from build123d import *

# Parameters (mm, degrees)
SKETCH_1_W          = 20
SKETCH_1_H          = 10.24
EXTRUDE_1_DEPTH     = 6.5
SKETCH_2_R          = 1.25
CUT_EXTRUDE_1_DEPTH = 7.5
SKETCH_4_W          = 2.303604444
SKETCH_4_H          = 2.775905185
EXTRUDE_2_DEPTH     = 8


with BuildPart() as part:
    # 草图1 → 凸台-拉伸1 (new body)
    with BuildSketch(Plane(origin=(0, 0, 0), x_dir=(1, 0, 0), z_dir=(0, 1, 0))):
        Rectangle(SKETCH_1_W, SKETCH_1_H)
    extrude(amount=EXTRUDE_1_DEPTH)

    # 草图2 → 切除-拉伸1 (cut, through all)
    with BuildSketch(Plane(origin=(0, 6.5, 0), x_dir=(1, 0, 0), z_dir=(0, 1, 0))):
        with Locations((-4.75, -2.62)):
            Circle(SKETCH_2_R)
        with Locations((4.75, -2.62)):
            Circle(SKETCH_2_R)
    extrude(amount=-CUT_EXTRUDE_1_DEPTH, mode=Mode.SUBTRACT)

    # 草图4 → 凸台-拉伸2 (add)
    with BuildSketch(Plane(origin=(0, 0, -5.12), x_dir=(-1, 0, 0), z_dir=(0, 0, -1))):
        with Locations((8.848197778, 3.213855402)):
            Rectangle(SKETCH_4_W, SKETCH_4_H)
    extrude(amount=EXTRUDE_2_DEPTH)


solid = part.part
Could you check a few things on this model? Use its own coordinates, in mm. A direction names the side the tool comes from. Coordinates: 2 decimals unless noted, no trailing zeros. Loops run counter-clockwise (first coordinate to the right, second up) from the corner with the lowest first, then second, coordinate; pieces in that order, holes last.
1. Imagine slicing it at A-A (x = -5.5). Please give me the cut outline in (y, z), and give its area (3 significant figures).
2. Imagine slicing it at B-B (z = 2.62). Please give me the cut outline in (x, y).
3. Imagine slicing it at D-D (x = 4.75). Please give me the cut outline in (y, z).
4. Imagine slicing it at C-C (y = 4). Please give me the cut outline in (x, z).
5. For faces 5 (the face through (-9, 4.602, -9)), 6 (the face through (-9, 1.826, -9)), 7 (the face through (-5.74, 3.3, 3.38)), 8 (the face through (-7.696, 3, -9)), which set-ups out of +Z, -Z, +X, -X, +Y, -Y let a thin tool reach every point of the face, with its end or its side?
6. We'd pull the mould along Z, two halves only. Please class faces 1 (the face through (4.48, 3.3, 3.84)), 2 (the face through (0, 3, 5.12)), 3 (the face through (0, 0, 0)), 4 (the face through (-9, 3, -13.12)): released by +Z, released by -Z, zero draft, split by the parting line, or undercut.
7. For P1, Ø1.5, axis at x = -2.5, y = 1, coming from the -Z side; P2, Ø0.8, axis at y = 3.5, z = -10, coming from the +X side; P3, Ø2.5, axis at x = -9, z = -9.5, coming from the -Y side, each with a flat end and sliding along its axis, tell me the tip position at first contact or that it passes through.
8. I need wall thicknesses on L1, parallel to X at y = 3.75, z = 2.62; L2, parallel to Z at x = 4.75, y = 2; L3, parallel to Z at x = 8.5, y = 1. Which ranges of each line are inside material? Lowest first, please.
Computed values:
1. outline: (0, -5.12) - (6.5, -5.12) - (6.5, 1.62) - (0, 1.62) - close; (0, 3.62) - (6.5, 3.62) - (6.5, 5.12) - (0, 5.12) - close
1. area: 53.6 mm2
2. outline: (-10, 0) - (-6, 0) - (-6, 6.5) - (-10, 6.5) - close; (-3.5, 0) - (3.5, 0) - (3.5, 6.5) - (-3.5, 6.5) - close; (6, 0) - (10, 0) - (10, 6.5) - (6, 6.5) - close
3. outline: (0, -5.12) - (6.5, -5.12) - (6.5, 1.37) - (0, 1.37) - close; (0, 3.87) - (6.5, 3.87) - (6.5, 5.12) - (0, 5.12) - close
4. outline: (-10, -13.12) - (-7.7, -13.12) - (-7.7, -5.12) - (10, -5.12) - (10, 5.12) - (-10, 5.12) - close; hole circle Ø2.5 at (-4.75, 2.62); hole circle Ø2.5 at (4.75, 2.62)
5. face 5: -Z, +X, -X, +Y
5. face 6: -Z, +X, -X, -Y
5. face 7: +Y, -Y
5. face 8: -Z, +X, +Y, -Y
6. face 1: undercut
6. face 2: released by +Z
6. face 3: zero draft
6. face 4: released by -Z
7. P1: stops at z = -5.12
7. P2: stops at x = -7.7
7. P3: stops at y = 1.83
8. L1: x = -10 to -6, -3.5 to 3.5, 6 to 10
8. L2: z = -5.12 to 1.37, 3.87 to 5.12
8. L3: z = -5.12 to 5.12
